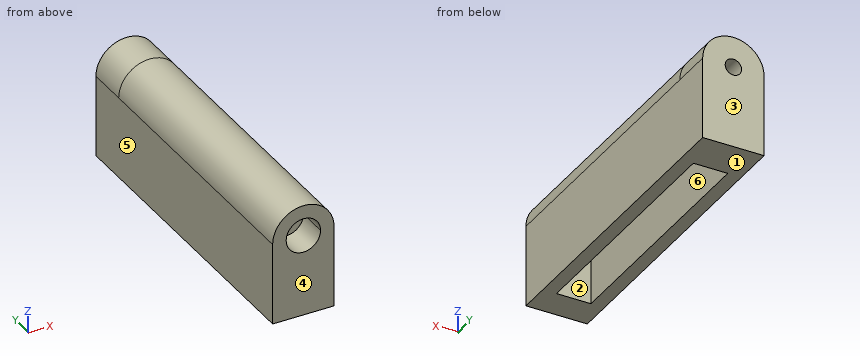
from build123d import *

# Parameters (mm, degrees)
F1_DEPTH = 19.05
F2_DEPTH = 152.4
F3_R     = 10.668
F3_R_2   = 5.08
F4_DEPTH = 25.4


with BuildPart() as f1:
    # F0 (on Front) → F1 (new body)
    with BuildSketch(Plane.XZ):
        with BuildLine():
            Line((19.05, -50.8), (19.05, 0))
            ThreePointArc((19.05, 0), (18.8393338746, 2.8252432042), (18.2119948386, 5.588))
            Line((18.2119948386, 5.588), (10.668, 5.588))
            Line((10.668, 5.588), (10.668, 0))
            Line((10.668, 0), (10.668, -50.8))
            Line((10.668, -50.8), (19.05, -50.8))
        make_face()
        with BuildLine():
            Line((10.668, 5.588), (18.2119948386, 5.588))
            ThreePointArc((18.2119948386, 5.588), (0, 19.05), (-18.2119948386, 5.588))
            Line((-18.2119948386, 5.588), (-10.668, 5.588))
            Line((-10.668, 5.588), (-9.0873802606, 5.588))
            ThreePointArc((-9.0873802606, 5.588), (0, 10.668), (9.0873802606, 5.588))
            Line((9.0873802606, 5.588), (10.668, 5.588))
        make_face()
        with BuildLine():
            Line((-10.668, 5.588), (-18.2119948386, 5.588))
            ThreePointArc((-18.2119948386, 5.588), (-18.8393338746, 2.8252432042), (-19.05, 0))
            Line((-19.05, 0), (-19.05, -50.8))
            Line((-19.05, -50.8), (-10.668, -50.8))
            Line((-10.668, -50.8), (-10.668, 0))
            Line((-10.668, 0), (-10.668, 5.588))
        make_face()
        with BuildLine():
            Line((-10.668, -50.8), (10.668, -50.8))
            Line((10.668, -50.8), (10.668, 0))
            ThreePointArc((10.668, 0), (0, -10.668), (-10.668, 0))
            Line((-10.668, 0), (-10.668, -50.8))
        make_face()
        with BuildLine():
            Line((10.668, 0), (10.668, 5.588))
            Line((10.668, 5.588), (9.0873802606, 5.588))
            ThreePointArc((9.0873802606, 5.588), (10.2652422431, 2.9036228561), (10.668, 0))
        make_face()
        with BuildLine():
            Line((-9.0873802606, 5.588), (-10.668, 5.588))
            Line((-10.668, 5.588), (-10.668, 0))
            ThreePointArc((-10.668, 0), (-10.2652422431, 2.9036228561), (-9.0873802606, 5.588))
        make_face()
    extrude(amount=F1_DEPTH)

    # F0 (on Front) → F2 (join)
    with BuildSketch(Plane.XZ):
        with BuildLine():
            Line((19.05, -50.8), (19.05, 0))
            ThreePointArc((19.05, 0), (18.8393338746, 2.8252432042), (18.2119948386, 5.588))
            Line((18.2119948386, 5.588), (10.668, 5.588))
            Line((10.668, 5.588), (10.668, 0))
            Line((10.668, 0), (10.668, -50.8))
            Line((10.668, -50.8), (19.05, -50.8))
        make_face()
        with BuildLine():
            Line((10.668, 5.588), (18.2119948386, 5.588))
            ThreePointArc((18.2119948386, 5.588), (0, 19.05), (-18.2119948386, 5.588))
            Line((-18.2119948386, 5.588), (-10.668, 5.588))
            Line((-10.668, 5.588), (-9.0873802606, 5.588))
            ThreePointArc((-9.0873802606, 5.588), (0, 10.668), (9.0873802606, 5.588))
            Line((9.0873802606, 5.588), (10.668, 5.588))
        make_face()
        with BuildLine():
            Line((-10.668, 5.588), (-18.2119948386, 5.588))
            ThreePointArc((-18.2119948386, 5.588), (-18.8393338746, 2.8252432042), (-19.05, 0))
            Line((-19.05, 0), (-19.05, -50.8))
            Line((-19.05, -50.8), (-10.668, -50.8))
            Line((-10.668, -50.8), (-10.668, 0))
            Line((-10.668, 0), (-10.668, 5.588))
        make_face()
    extrude(amount=-F2_DEPTH)

    # F3 (on face) → F4 (join)
    with BuildSketch(Plane(origin=(0, 152.4, 0), x_dir=(-1, 0, 0), z_dir=(0, 1, 0))):
        with BuildLine():
            ThreePointArc((19.05, 0), (0, 19.05), (-19.05, 0))
            Line((-19.05, 0), (-19.05, -50.8))
            Line((-19.05, -50.8), (19.05, -50.8))
            Line((19.05, -50.8), (19.05, 0))
        make_face()
        Circle(F3_R, mode=Mode.SUBTRACT)
        with BuildLine():
            ThreePointArc((-9.0873802606, 5.588), (-10.2652422431, 2.903622856), (-10.668, -1e-10))
            ThreePointArc((-10.668, -1e-10), (0, -10.668), (10.668, 0))
            ThreePointArc((10.668, 0), (10.2652422431, 2.9036228561), (9.0873802606, 5.588))
            ThreePointArc((9.0873802606, 5.588), (0, 10.668), (-9.0873802606, 5.588))
        make_face()
        Circle(F3_R_2, mode=Mode.SUBTRACT)
    extrude(amount=F4_DEPTH)


solid = f1.part
Can you work these out from the model? Positions are in its coordinate system, mm. Face numbers are marked on the shaded views. A direction names the side the tool comes from. Give positions to 0.01 mm unless a question says otherwise; leave off trailing zeros. Order: outer loops, then holes, each group sorted by start corner. A loop starts at its lowest first (then second) coordinate and runs counter-clockwise, first axis right, second up. Notation, with made-up numbers: M 40.5,7.25 L 85.5,7.25 A33 ccw 85.5,44.25 Z; hole C 35.25,4.5 d11. An arc over 180 degrees is marked long. Use a Markdown table: item, result. Add a question column.
Item 1: Suppose I cut it at C-C (y = 28.5). List the corners of the cut face in (x, z) for me, then the cut area to 3 significant figures.
Item 2: Suppose I cut it at D-D (y = 165.5). List the corners of the cut face in (x, z) for me, then the cut area to 3 significant figures.
Item 3: Will these pins go through, and if not, where does the flat tip stop? pin 1 (5 mm diameter, centred on x = 4.5, z = 9, fed in from -Y); pin 2 (6 mm diameter, centred on x = 4, y = 117, fed in from +Z); pin 3 (1 mm diameter, centred on x = 6, y = 42, fed in from -Z); pin 4 (1.3 mm diameter, centred on x = 9.5, y = 77, fed in from -Z).
Item 4: We'd pull the mould along Y, two halves only. Please class the marked faces 3, 4, 5 and 6: +Y half, -Y half, draft (parallel to the pull), parting line (faces both ways), or undercut.
Item 5: If I drill on L1, parallel to X at y = 92.5, z = -44.5; L2, parallel to Y at x = 2, z = -40.5; L3, parallel to Z at x = 0, y = 160, over which ranges is the centre line in solid material (lowest first)? Write a range as [from, to].
Item 6: Suppose I cut it at B-B (z = -33). List the corners of the cut face in (x, y) for me.
Item 7: Suppose I cut it at A-A (x = 0). List the corners of the cut face in (y, z) for me.
Item 8: For the marked faces 1 and 2, which set-ups out of +Z, -Z, +X, -X, +Y, -Y let a thin tool reach every point of the face, with its end or its side?
Answer sheet:
| question | item | result |
|---|---|---|
| 1 | outline | M -19.05,-50.8 L -10.67,-50.8 L -10.67,5.59 L -9.09,5.59 A10.67 cw 9.09,5.59 L 10.67,5.59 L 10.67,-50.8 L 19.05,-50.8 L 19.05,0 A19.05 ccw -19.05,0 Z |
| 1 | area | 1,240 mm² |
| 2 | outline | M -19.05,-50.8 L 19.05,-50.8 L 19.05,0 A19.05 ccw -19.05,0 Z; hole C 0,0 d10.16 |
| 2 | area | 2,420 mm² |
| 3 | pin 1 | stops at y = -19.05 |
| 3 | pin 2 | stops at z = 19.02 |
| 3 | pin 3 | stops at z = 8.46 |
| 3 | pin 4 | stops at z = 5.59 |
| 4 | face 3 | +Y half |
| 4 | face 4 | -Y half |
| 4 | face 5 | draft |
| 4 | face 6 | undercut |
| 5 | L1 | x = [-19.05, -10.67], [10.67, 19.05] |
| 5 | L2 | y = [-19.05, 0], [152.4, 177.8] |
| 5 | L3 | z = [-50.8, -5.08], [5.08, 19.05] |
| 6 | outline | M -19.05,-19.05 L 19.05,-19.05 L 19.05,177.8 L -19.05,177.8 Z; hole M -10.67,0 L 10.67,0 L 10.67,152.4 L -10.67,152.4 Z |
| 7 | outline | M -19.05,-50.8 L 0,-50.8 L 0,-10.67 L -19.05,-10.67 Z; M -19.05,10.67 L 152.4,10.67 L 152.4,5.08 L 177.8,5.08 L 177.8,19.05 L -19.05,19.05 Z; M 152.4,-50.8 L 177.8,-50.8 L 177.8,-5.08 L 152.4,-5.08 Z |
| 8 | face 1 | -Z, +X, -X, +Y, -Y |
| 8 | face 2 | -Z |
